Check sheet for the modelled part. Datum: model origin and axes. Units: mm. Round coordinates to 2 decimals unless told otherwise and drop trailing zeros. Write each loop counter-clockwise with the first axis right and the second up, starting at its lowest first coordinate (ties: lowest second). Pieces come first, ordered by that corner, then holes. Notation, with made-up numbers: M 74.5,55 L 104.5,55 A18 ccw 104.5,69 Z; hole C -24,11.5 d1. An arc over 180 degrees is marked long. Answer in a Markdown table with one row per item.
```python
from build123d import *

# Parameters (mm, degrees)
SKETCH_1_W      = 16
SKETCH_1_H      = 8.7
EXTRUDE_1_DEPTH = 3
CHAMFER_3_SIZE  = 2
CHAMFER_4_SIZE  = 0.3


with BuildPart() as part:
    # Эскиз1 → Вытянуть1 (new body)
    with BuildSketch(Plane.XY):
        with Locations((8, 4.35)):
            Rectangle(SKETCH_1_W, SKETCH_1_H)
    extrude(amount=EXTRUDE_1_DEPTH)

    # Фаска3
    chamfer_3_edges = [part.edges().sort_by_distance(p)[0] for p in [
        (8, 0, 3),
    ]]
    chamfer(chamfer_3_edges, length=CHAMFER_3_SIZE)

    # Фаска4
    chamfer_4_edges = [part.edges().sort_by_distance(p)[0] for p in [
        (16, 0, 0.5),
    ]]
    chamfer(chamfer_4_edges, length=CHAMFER_4_SIZE)


solid = part.part
```
1. Section check A-A, the plane x = 12.25. Record the cut outline in (y, z), and give its area (3 significant figures).
Found:
| item | result |
|---|---|
| outline | M 0,0 L 8.7,0 L 8.7,3 L 2,3 L 0,1 Z |
| area | 24.1 mm2 |
2. Section check B-B, the plane z = 2. Record the cut outline in (x, y).
Found:
| item | result |
|---|---|
| outline | M 0,1 L 16,1 L 16,8.7 L 0,8.7 Z |
3. Scan lines: L1, parallel to Y at x = 10.75, z = 2.25; L2, parallel to Z at x = 10.25, y = 1.5; L3, parallel to Z at x = 15, y = 1. Record each from-to range of solid material in increasing order.
Found:
| item | result |
|---|---|
| L1 | y = 1.25 to 8.7 |
| L2 | z = 0 to 2.5 |
| L3 | z = 0 to 2 |
4. Section check C-C, the plane z = 2.75. Record the cut outline in (x, y), and give its area (3 significant figures).
Found:
| item | result |
|---|---|
| outline | M 0,1.75 L 16,1.75 L 16,8.7 L 0,8.7 Z |
| area | 111 mm2 |
